from build123d import *

# Parameters (mm, degrees)
SKETCH1_W                                        = 152.4
SKETCH1_H                                        = 101.6
BOSS_EXTRUDE1_DEPTH                              = 12.7
CBORE_FOR_1_4_SOCKET_HEAD_CAP_SCREW1_D           = 7.14248
CBORE_FOR_1_4_SOCKET_HEAD_CAP_SCREW1_CBORE_D     = 11.1125
CBORE_FOR_1_4_SOCKET_HEAD_CAP_SCREW1_CBORE_DEPTH = 8.89
TAP_DRILL_FOR_1_4_20_TAP1_D                      = 5.1054


with BuildPart() as part:
    # Sketch1 → Boss-Extrude1 (new body)
    with BuildSketch(Plane(origin=(0, 0, 0), x_dir=(1, 0, 0), z_dir=(0, 1, 0))):
        Rectangle(SKETCH1_W, SKETCH1_H)
    extrude(amount=BOSS_EXTRUDE1_DEPTH)

    # CBORE for 1/4 Socket Head Cap Screw1 (through all)
    with Locations(Plane(origin=(0, 12.7, 0), x_dir=(1, 0, 0), z_dir=(0, 1, 0))):
        with Locations((-38.1, 38.1), (38.1, 38.1), (38.1, -38.1), (-38.1, -38.1)):
            CounterBoreHole(CBORE_FOR_1_4_SOCKET_HEAD_CAP_SCREW1_D / 2, CBORE_FOR_1_4_SOCKET_HEAD_CAP_SCREW1_CBORE_D / 2, CBORE_FOR_1_4_SOCKET_HEAD_CAP_SCREW1_CBORE_DEPTH)

    # Tap Drill for 1/4-20 Tap1 (through all)
    with Locations(Plane(origin=(0, 12.7, 0), x_dir=(1, 0, 0), z_dir=(0, 1, 0))):
        with Locations((0, 0), (25.4, 0), (50.8, 0), (-25.4, 0), (-50.8, 0)):
            Hole(TAP_DRILL_FOR_1_4_20_TAP1_D / 2)


solid = part.part
Verification items for the finished model (mm, model axes). A direction names the side the tool comes from. Coordinates: 2 decimals unless noted, no trailing zeros. Order: outer loops, then holes, each group sorted by start corner. A loop starts at its lowest first (then second) coordinate and runs counter-clockwise, first axis right, second up. Notation, with made-up numbers: M 21.25,36 L 78.25,36 A15 cw 78.25,46 Z; hole C 64.25,35 d2. An arc over 180 degrees is marked long. Write each question's results on one line, items separated by ' | '.
1) Section check B-B on y = 5.5. Give the number of separate pieces and of enclosed holes in the cut face, plus the area to 3 significant figures.
Solved:
separate pieces: 1 | enclosed holes: 9 | area: 15,000 mm²
2) Release check for a two-part mould opening along Z. For faces 3 (the face through (41.668, 1.878, 37.943)), 4 (the face through (-1, 12.7, 11)), 5 (the face through (-1, 6, -50.8)) record: pulls with the +Z half, pulls with the -Z half, needs draft (parallel to the pull), parting line crosses it, or undercut.
Solved:
face 3: undercut | face 4: needs draft | face 5: pulls with the -Z half
3) Section check D-D on z = 0. Record the cut outline in (x, y).
Solved:
outline: M -76.2,0 L -53.35,0 L -53.35,12.7 L -76.2,12.7 Z; M -48.25,0 L -27.95,0 L -27.95,12.7 L -48.25,12.7 Z; M -22.85,0 L -2.55,0 L -2.55,12.7 L -22.85,12.7 Z; M 2.55,0 L 22.85,0 L 22.85,12.7 L 2.55,12.7 Z; M 27.95,0 L 48.25,0 L 48.25,12.7 L 27.95,12.7 Z; M 53.35,0 L 76.2,0 L 76.2,12.7 L 53.35,12.7 Z
4) Access from +Z, -Z, +X, -X, +Y, -Y to the whole of each face (thin tool, end or side, straight path). Record for faces 1 (the face through (41.087, 8.317, -42.785)), 2 (the face through (-39.748, 1.878, -34.932)).
Solved:
face 1: +Y | face 2: +Y, -Y
5) Section check A-A on z = 38.1. Record the cut outline in (x, y).
Solved:
outline: M -76.2,0 L -41.67,0 L -41.67,3.81 L -43.66,3.81 L -43.66,12.7 L -76.2,12.7 Z; M -34.53,0 L 34.53,0 L 34.53,3.81 L 32.54,3.81 L 32.54,12.7 L -32.54,12.7 L -32.54,3.81 L -34.53,3.81 Z; M 41.67,0 L 76.2,0 L 76.2,12.7 L 43.66,12.7 L 43.66,3.81 L 41.67,3.81 Z
6) Section check C-C on x = 50.8. Record the cut outline in (y, z).
Solved:
outline: M 0,-50.8 L 12.7,-50.8 L 12.7,-2.55 L 0,-2.55 Z; M 0,2.55 L 12.7,2.55 L 12.7,50.8 L 0,50.8 Z
7) Scan lines: line 1 along X through (y, z) = (9.25, 38.1); line 2 along X through (y, z) = (2.1, -38.1); line 3 along Z through (x, y) = (-38.1, 1.15). Record each from-to range of solid material in increasing order. Write a range as [from, to].
Solved:
line 1: x = [-76.2, -43.66], [-32.54, 32.54], [43.66, 76.2] | line 2: x = [-76.2, -41.67], [-34.53, 34.53], [41.67, 76.2] | line 3: z = [-50.8, -41.67], [-34.53, 34.53], [41.67, 50.8]
8) Gauge pin test, flat ends, axial feed: pin 1 Ø6.5 at (x, z) = (-38.1, -38.1) entering from -Y; pin 2 Ø9 at (x, z) = (38.1, -38.1) entering from +Y. Record the tip position at first contact, or that the pin passes through.
Solved:
pin 1: passes through | pin 2: stops at y = 3.81
